Can you work these out from the model? Positions are in its coordinate system, mm. Face numbers are marked on the shaded views. Coordinates: 2 decimals unless noted, no trailing zeros. Loops run counter-clockwise (first coordinate to the right, second up) from the corner with the lowest first, then second, coordinate; pieces in that order, holes last. Notation, with made-up numbers: M 12,-20 L 38,-20 A17 cw 38,3 Z; hole C 33,29.25 d3. An arc over 180 degrees is marked long. Answer as a JSON object with one key per item and string values. Group by question number.
Item 1: Suppose I cut it at C-C (x = 5). Write out the boundary of the cut face in (y, z), then the cut area to 3 significant figures.
Item 2: If I drill on line 1 (Y direction, x = 0, z = 3.35); line 2 (Y direction, x = 5, z = 1.8); line 3 (X direction, y = -0.5, z = 2.55), over which ranges is the centre line in solid material (lowest first)?
Item 3: We'd pull the mould along X, two halves only. Please class the marked faces 1, 2 and 3: +X half, -X half, draft (parallel to the pull), parting line (faces both ways), or undercut.
Item 4: Suppose I cut it at D-D (y = 0). Write out the boundary of the cut face in (x, z), then the cut area to 3 significant figures.
Item 5: Suppose I cut it at B-B (z = 1.6). Write out the boundary of the cut face in (x, y).
Item 6: I'm going to push a flat-ended pin straight in: pin 1 Ø10 at (x, y) = (0.5, -6) entering from -Z. Where does the tip first touch, or does it pass through?
Item 7: Suppose I cut it at A-A (y = -5). Write out the boundary of the cut face in (x, z), then the cut area to 3 significant figures.
```python
from build123d import *

# Parameters (mm, degrees)
SKETCH_1_W          = 20
SKETCH_1_H          = 20
SKETCH_1_R          = 1.5
EXTRUDE_1_DEPTH     = 5
SKETCH_2_R          = 1.5
CUT_EXTRUDE_1_DEPTH = 10


with BuildPart() as part:
    # 草图1 → 凸台-拉伸1 (new body)
    with BuildSketch(Plane.XY):
        Rectangle(SKETCH_1_W, SKETCH_1_H)
        Circle(SKETCH_1_R, mode=Mode.SUBTRACT)
    extrude(amount=EXTRUDE_1_DEPTH)

    # 草图2 → 切除-拉伸1 (cut)
    with BuildSketch(Plane.XY.offset(5)):
        with Locations((-5, -5)):
            Circle(SKETCH_2_R)
        with Locations((5, -5)):
            Circle(SKETCH_2_R)
    extrude(amount=-CUT_EXTRUDE_1_DEPTH, mode=Mode.SUBTRACT)


solid = part.part
```
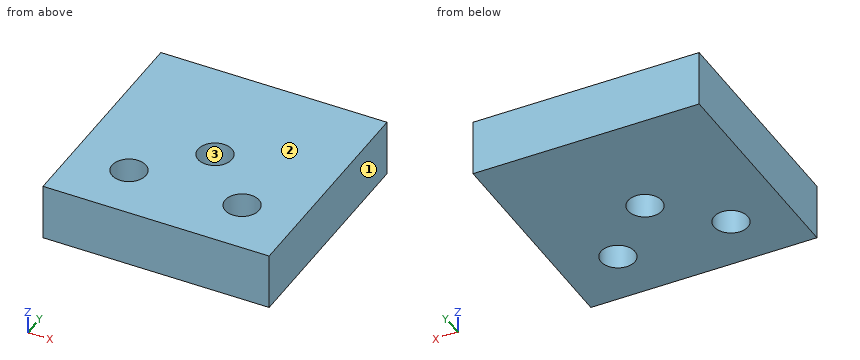
From the geometry:
{
 "1": {"outline": "M -10,0 L -6.5,0 L -6.5,5 L -10,5 Z; M -3.5,0 L 10,0 L 10,5 L -3.5,5 Z", "area": "85.0 mm2"},
 "2": {"line 1": "-10 to -1.5, 1.5 to 10", "line 2": "-10 to -6.5, -3.5 to 10", "line 3": "-10 to -1.41, 1.41 to 10"},
 "3": {"face 1": "+X half", "face 2": "draft", "face 3": "undercut"},
 "4": {"outline": "M -10,0 L -1.5,0 L -1.5,5 L -10,5 Z; M 1.5,0 L 10,0 L 10,5 L 1.5,5 Z", "area": "85.0 mm2"},
 "5": {"outline": "M -10,-10 L 10,-10 L 10,10 L -10,10 Z; hole C -5,-5 d3; hole C 0,0 d3; hole C 5,-5 d3"},
 "6": {"pin 1": "z = 0"},
 "7": {"outline": "M -10,0 L -6.5,0 L -6.5,5 L -10,5 Z; M -3.5,0 L 3.5,0 L 3.5,5 L -3.5,5 Z; M 6.5,0 L 10,0 L 10,5 L 6.5,5 Z", "area": "70.0 mm2"}
}
